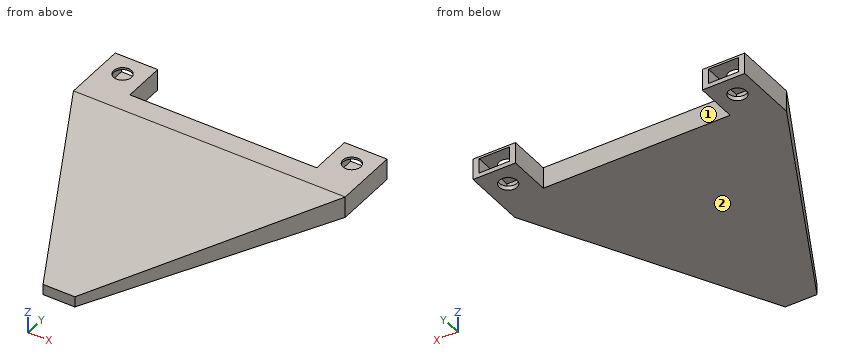
```python
from build123d import *

# Parameters (mm, degrees)
SKETCH002_W  = 128
SKETCH002_H  = 10
SKETCH001_W  = 15
SKETCH001_H  = 5
SKETCH_R     = 4.2
PAD_DEPTH    = 10
SKETCH003_W  = 14.2
SKETCH003_H  = 7
POCKET_DEPTH = 20


with BuildPart() as loft_body:
    # Sketch002 → Loft section 0
    with BuildSketch(Plane.XZ):
        with Locations((0, 5)):
            Rectangle(SKETCH002_W, SKETCH002_H)
    # Sketch001 → Loft section 1
    with BuildSketch(Plane.XZ.offset(108)):
        with Locations((0, 2.5)):
            Rectangle(SKETCH001_W, SKETCH001_H)
    loft()


with BuildPart() as pocket:
    # Sketch → Pad (new body)
    with BuildSketch(Plane.XY):
        Polygon((-64, 30), (-64, 0), (64, 0), (64, 30), (44, 30), (44, 10), (-44, 10), (-44, 30), align=None)
        with Locations((-54, 20)):
            Circle(SKETCH_R, mode=Mode.SUBTRACT)
        with Locations((54, 20)):
            Circle(SKETCH_R, mode=Mode.SUBTRACT)
    extrude(amount=PAD_DEPTH)

    # Fusion: union Loft body
    add(loft_body.part)

    # Sketch003 → Pocket (cut)
    with BuildSketch(Plane(origin=(0, 30, 0), x_dir=(-1, 0, 0), z_dir=(0, 1, 0))):
        with Locations((54, 5.5)):
            Rectangle(SKETCH003_W, SKETCH003_H)
        with Locations((-54, 5.5)):
            Rectangle(SKETCH003_W, SKETCH003_H)
    extrude(amount=-POCKET_DEPTH, mode=Mode.SUBTRACT)


solid = pocket.part
```
For this review, take the finished solid that the model builds, in its own axes (mm). Face numbers are marked on the shaded views. A direction names the side the tool comes from. Round coordinates to 2 decimals unless told otherwise and drop trailing zeros. One line per item, written item: value. Start each with the question number.
(1) Insertion check: pin 1 (3 mm diameter, centred on x = -19.5, z = 8, fed in from +Y); pin 2 (5 mm diameter, centred on x = -54, y = 20, fed in from +Z); pin 3 (4 mm diameter, centred on x = -14, y = -61, fed in from +Z); pin 4 (1 mm diameter, centred on x = 35, z = 4, fed in from -Y). Each pin has a flat end and moves straight along its axis. Give the tip position at first contact, or say it passes through.
(2) We need section A-A (x = -54). Count the separate pieces of the cut face and the enclosed holes in it, and give its area (3 significant figures).
(3) Wall thickness on line 1 (X direction, y = 20, z = 9.85); line 2 (Z direction, x = 5.5, y = -21.5); line 3 (X direction, y = -44.5, z = 4.75): over which ranges is each line inside the solid? List them lowest first.
(4) Machinability: for the marked faces 1 and 2, which of the approach directions +Z, -Z, +X, -X, +Y, -Y give a long, thin tool a straight path to every point of the face, cutting with its end or side? Answer none if there is none.
Result:
1. pin 1: y = 10
1. pin 2: through
1. pin 3: z = 7.27
1. pin 4: y = -56.39
2. separate pieces: 3
2. enclosed holes: 0
2. area: 317 mm²
3. line 1: -64 to -58.2, -49.8 to -44, 44 to 49.8, 58.2 to 64
3. line 2: 0 to 9
3. line 3: -40.72 to 40.72
4. face 1: +Z, -Z, +Y
4. face 2: -Z, +X, -X, +Y, -Y
